Read the model definition and answer for the solid it produces. Units are mm, in the model's axes. Face numbers are marked on the shaded views. Coordinates: 2 decimals unless noted, no trailing zeros. Loops run counter-clockwise (first coordinate to the right, second up) from the corner with the lowest first, then second, coordinate; pieces in that order, holes last.
from build123d import *

# Parameters (mm, degrees)
BOSS_EXTRUDE2_DEPTH      = 3
BOSS_EXTRUDE2_DEPTH_BACK = 109.6
SKETCH3_R                = 333
SKETCH3_R_2              = 330
SKETCH5_R                = 330
BOSS_EXTRUDE4_DEPTH      = 3
SKETCH6_R                = 333
BOSS_EXTRUDE6_DEPTH      = 3
SKETCH17_R               = 330
BOSS_EXTRUDE9_DEPTH      = 3
CUT_EXTRUDE1_DEPTH       = 501.508020593
CUT_EXTRUDE1_DEPTH_BACK  = 501.508020593
SKETCH18_W               = 712.715925151
SKETCH18_H               = 346.222463294
SKETCH19_W               = 50
SKETCH19_H               = 10
SKETCH19_W_2             = 10
SKETCH19_H_2             = 50
SKETCH19_W_3             = 30
BOSS_EXTRUDE10_DEPTH     = 10
SKETCH20_W               = 1.85878785
SKETCH20_H               = 109.6
SKETCH20_W_2             = 1.900186503
CUT_EXTRUDE2_DEPTH       = 4.1
CUT_EXTRUDE3_START       = -11
SKETCH23_R               = 1.5
CUT_EXTRUDE3_DEPTH       = 11
SKETCH24_W               = 40
SKETCH24_H               = 144
CUT_EXTRUDE4_DEPTH       = 3
BOSS_EXTRUDE11_DEPTH     = 3


with BuildPart() as part:
    # Sketch3 → Boss-Extrude2 (new, two sides: drawn at the far end of the back side and taken through both)
    with BuildSketch(Plane(origin=(0, 0, 0), x_dir=(1, 0, 0), z_dir=(0, 1, 0)).offset(-BOSS_EXTRUDE2_DEPTH_BACK)):
        with Locations(Location((-11.008302555, 15.174390861, 0), (0, 0, 270))):
            Circle(SKETCH3_R)
        with Locations(Location((-11.008302555, 15.174390861, 0), (0, 0, 270))):
            Circle(SKETCH3_R_2, mode=Mode.SUBTRACT)
    extrude(amount=BOSS_EXTRUDE2_DEPTH + BOSS_EXTRUDE2_DEPTH_BACK)

    # Sketch5 → Boss-Extrude4 (add)
    with BuildSketch(Plane.XZ.offset(104.6)):
        with Locations(Location((-11.008302555, -15.174390861, 0), (0, 0, 90))):
            Circle(SKETCH5_R)
        with BuildLine():
            Line((-164.332788108, -283.060090014), (142.316182998, -283.060090014))
            ThreePointArc((142.316182998, -283.060090014), (-11.008302555, 293.485852256), (-164.332788108, -283.060090014))
        make_face(mode=Mode.SUBTRACT)
    extrude(amount=-BOSS_EXTRUDE4_DEPTH)

    # Sketch6 → Boss-Extrude6 (add)
    with BuildSketch(Plane(origin=(0, 0, 0), x_dir=(1, 0, 0), z_dir=(0, 1, 0))):
        with Locations(Location((-11.008302555, 15.174390861, 0), (0, 0, 270))):
            Circle(SKETCH6_R)
        Polygon((187.991697445, -189.598621739), (187.991697445, 20.401378261), (224.991697445, 20.401378261), (224.991697445, 100.970480915), (60.317326344, 288.174390861), (-82.333931455, 288.174390861), (-247.008302555, 100.970480915), (-247.008302555, 20.401378261), (-210.008302555, 20.401378261), (-210.008302555, -189.598621739), align=None, mode=Mode.SUBTRACT)
    extrude(amount=BOSS_EXTRUDE6_DEPTH)

    # Sketch17 → Boss-Extrude9 (add)
    with BuildSketch(Plane(origin=(0, -5, 0), x_dir=(1, 0, 0), z_dir=(0, 1, 0))):
        with Locations(Location((-11.008302555, 15.174390861, 0), (0, 0, 270))):
            Circle(SKETCH17_R)
        with BuildLine():
            Line((142.316182998, 283.060090014), (-164.332788108, 283.060090014))
            ThreePointArc((-164.332788108, 283.060090014), (-11.008302555, -293.485852256), (142.316182998, 283.060090014))
        make_face(mode=Mode.SUBTRACT)
    extrude(amount=-BOSS_EXTRUDE9_DEPTH)

    # Sketch18 → Cut-Extrude1 (cut, two sides: drawn at the far end of the back side and taken through both)
    with BuildSketch(Plane(origin=(0, -5, 0), x_dir=(1, 0, 0), z_dir=(0, 1, 0)).offset(-CUT_EXTRUDE1_DEPTH_BACK)):
        with Locations((-7.081493051, 193.512609908)):
            Rectangle(SKETCH18_W, SKETCH18_H)
    extrude(amount=CUT_EXTRUDE1_DEPTH + CUT_EXTRUDE1_DEPTH_BACK, mode=Mode.SUBTRACT)

    # Sketch19 → Boss-Extrude10 (add)
    with BuildSketch(Plane(origin=(0, 3, 0), x_dir=(1, 0, 0), z_dir=(0, 1, 0))):
        with Locations((-185.008302555, -197.798621739)):
            Rectangle(SKETCH19_W, SKETCH19_H)
        with Locations((162.991697445, -197.798621739)):
            Rectangle(SKETCH19_W, SKETCH19_H)
        with Locations((196.191697445, -7.798621739)):
            Rectangle(SKETCH19_W_2, SKETCH19_H_2)
        with Locations((216.191697445, 12.201378261)):
            Rectangle(SKETCH19_W_3, SKETCH19_H)
        with Locations((-238.208302555, 12.201378261)):
            Rectangle(SKETCH19_W_3, SKETCH19_H)
        with Locations((-218.208302555, -7.798621739)):
            Rectangle(SKETCH19_W_2, SKETCH19_H_2)
    extrude(amount=BOSS_EXTRUDE10_DEPTH)

    # Sketch20 → Cut-Extrude2 (cut)
    with BuildSketch(Plane(origin=(0, 0, -20.401378261), x_dir=(-1, 0, 0), z_dir=(0, 0, -1))):
        with Locations((-319.72109137, -54.8)):
            Rectangle(SKETCH20_W, SKETCH20_H)
        with Locations((341.716997154, -54.8)):
            Rectangle(SKETCH20_W_2, SKETCH20_H)
    extrude(amount=-CUT_EXTRUDE2_DEPTH, mode=Mode.SUBTRACT)

    # Sketch23 → Cut-Extrude3 (cut)
    with BuildSketch(Plane(origin=(0, 3, 0), x_dir=(1, 0, 0), z_dir=(0, 1, 0)).offset(CUT_EXTRUDE3_START)):
        with Locations(Location((-266.430595358, -167.218017294, 0), (0, 0, 270))):
            Circle(SKETCH23_R)
        with Locations(Location((-262.835878396, 11.878802847, 0), (0, 0, 270))):
            Circle(SKETCH23_R)
        with Locations(Location((240.383738856, 11.878802847, 0), (0, 0, 270))):
            Circle(SKETCH23_R)
        with Locations(Location((244.931055017, -167.7800562, 0), (0, 0, 270))):
            Circle(SKETCH23_R)
        with Locations(Location((-118.508302555, -197.879856977, 0), (0, 0, 270))):
            Circle(SKETCH23_R)
        with Locations(Location((96.491697445, -197.879856977, 0), (0, 0, 270))):
            Circle(SKETCH23_R)
    extrude(amount=CUT_EXTRUDE3_DEPTH, mode=Mode.SUBTRACT)

    # Sketch24 → Cut-Extrude4 (cut)
    with BuildSketch(Plane(origin=(0, 3, 0), x_dir=(1, 0, 0), z_dir=(0, 1, 0))):
        with Locations((-252.008302555, -74.598621739)):
            Rectangle(SKETCH24_W, SKETCH24_H)
        with Locations((229.991697445, -74.598621739)):
            Rectangle(SKETCH24_W, SKETCH24_H)
    extrude(amount=-CUT_EXTRUDE4_DEPTH, mode=Mode.SUBTRACT)

    # Sketch25 → Boss-Extrude11 (add)
    with BuildSketch(Plane.XZ):
        Polygon((-272.008302555, 149.598621739), (-272.008302555, 146.598621739), (-232.008302555, 146.598621739), (-232.008302555, 2.598621739), (-272.008302555, 2.598621739), (-272.008302555, -0.401378261), (-230.008302555, -0.401378261), (-230.008302555, 149.598621739), align=None)
        Polygon((249.991697445, 149.598621739), (207.991697445, 149.598621739), (207.991697445, -0.401378261), (249.991697445, -0.401378261), (249.991697445, 2.598621739), (209.991697445, 2.598621739), (209.991697445, 146.598621739), (249.991697445, 146.598621739), align=None)
    extrude(amount=BOSS_EXTRUDE11_DEPTH)


solid = part.part
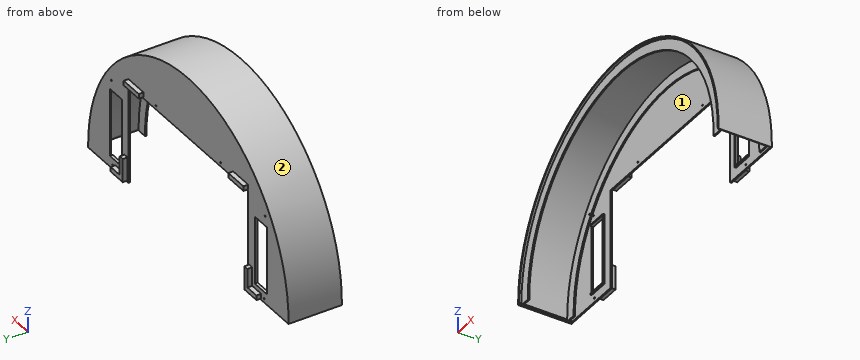
Item 1: Determine the mould class of the marked faces 1 and 2 for opening direction Y: released by +Y, released by -Y, zero draft, split by the parting line, or undercut.
Numbers:
face 1: undercut
face 2: zero draft
Item 2: Find the intervals of material crossed by line 1 along X through (y, z) = (-40, 235); line 2 along X through (y, z) = (-22.5, 23); line 3 along Y through (x, z) = (-76, 240.5), in increasing order.
Numbers:
line 1: x = -230.78 to -226.21, 204.2 to 208.77
line 2: x = -341.81 to -338.79, 316.78 to 319.8
line 3: y = 0 to 3
Item 3: Given pin 1 (5 mm diameter, centred on x = -266.43, z = 167.22, fed in from +Y); pin 2 (12 mm diameter, centred on y = -77.5, z = 198.5, fed in from -X); pin 3 (2.5 mm diameter, centred on x = -248.5, y = -2, fed in from +Z), each flat-ended and moving along its own axis, determine where each tip first touches the part or whether it passes through.
Numbers:
pin 1: stops at y = 3
pin 2: stops at x = -271.32
pin 3: stops at z = 219.51
Item 4: A cutting plane is placed at A-A on z = 159. Determine the outline of the cut face in (x, y), then the cut area to 3 significant figures.
Numbers:
outline: (-294.83, -109.6) - (-291.3, -109.6) - (-291.3, -104.6) - (-265.83, -104.6) - (-265.83, -101.6) - (-291.3, -101.6) - (-291.3, -8) - (-265.83, -8) - (-265.83, -5) - (-291.3, -5) - (-291.3, 0) - (-210.01, 0) - (-210.01, 3) - (-294.83, 3) - close; (187.99, 0) - (269.28, 0) - (269.28, -5) - (243.81, -5) - (243.81, -8) - (269.28, -8) - (269.28, -101.6) - (243.81, -101.6) - (243.81, -104.6) - (269.28, -104.6) - (269.28, -109.6) - (272.81, -109.6) - (272.81, 3) - (187.99, 3) - close
area: 1,590 mm2
Item 5: A cutting plane is placed at B-B on x = -98.5. Determine the outline of the cut face in (y, z).
Numbers:
outline: (-109.6, 303.02) - (-104.6, 303.02) - (-104.6, 280.83) - (-101.6, 280.83) - (-101.6, 303.02) - (-8, 303.02) - (-8, 280.83) - (-5, 280.83) - (-5, 303.02) - (0, 303.02) - (0, 189.6) - (3, 189.6) - (3, 306.13) - (-109.6, 306.13) - close
